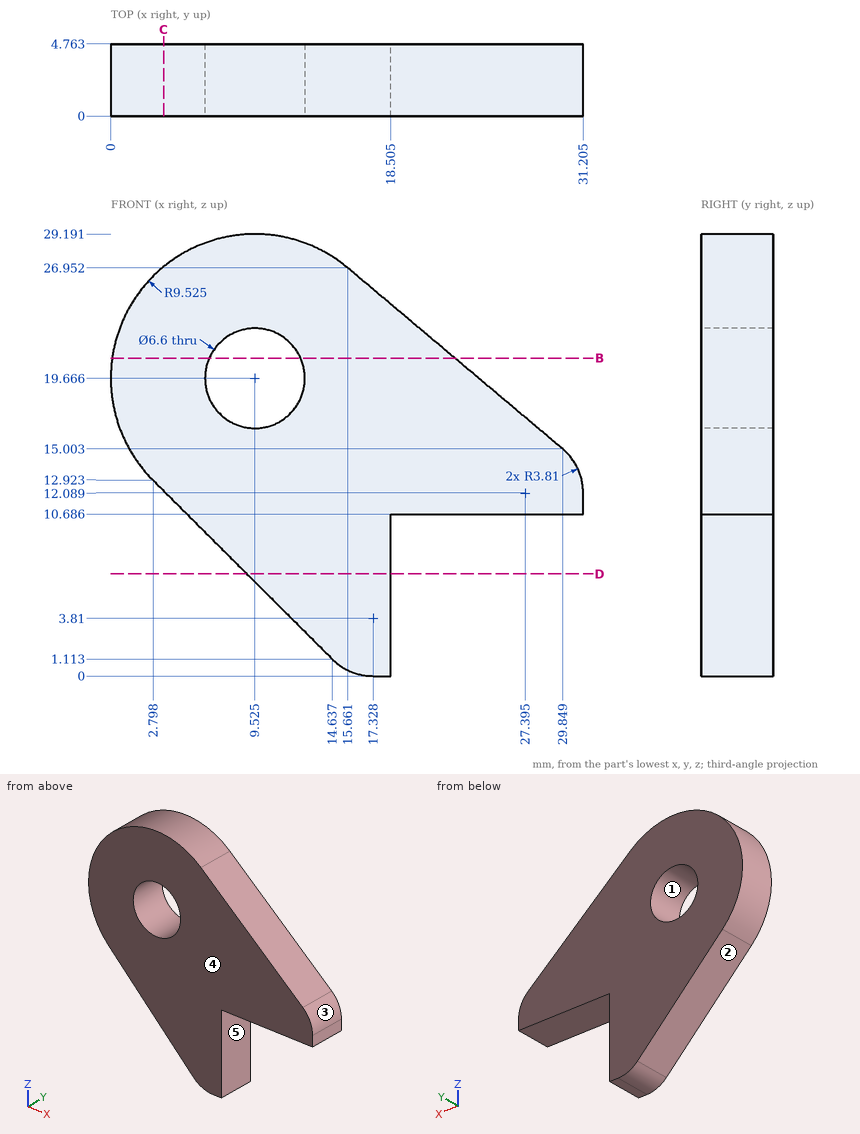
Input: dimensioned drawing with shaded views. Units: mm. Origin: part minimum x, y, z. A direction names the side the tool comes from. Coordinates: 2 decimals unless noted, no trailing zeros. Loops run counter-clockwise (first coordinate to the right, second up) from the corner with the lowest first, then second, coordinate; pieces in that order, holes last. Notation, with made-up numbers: M 89.5,30.25 L 116.5,30.25 A21 ccw 116.5,60.25 Z; hole C 86,-15.5 d9. An arc over 180 degrees is marked long. Use a Markdown table: item, result. Add a question column.
Q1. Section query C-C, the plane x = 3.5. Return loops of the section in (y, z).
Q2. Section query D-D, the plane z = 6.75. Return loops of the section in (x, y) (1 decimal).
Q3. First-contact query: pin 1 (4 mm diameter, centred on x = 9.52, z = 19.67, fed in from -Y); pin 2 (1.5 mm diameter, centred on y = 3, z = 18.5, fed in from -X); pin 3 (2 mm diameter, centred on y = 1.5, z = 11.5, fed in from -X); pin 4 (2.5 mm diameter, centred on x = 23, y = 3, fed in from -Z). Flat tips, straight axial feed; report the tip coordinate or a pass-through.
Q4. Section query B-B, the plane z = 21. Return loops of the section in (x, y).
Q5. Access query for the marked faces 4 and 5. Directions: +Z, -Z, +X, -X, +Y, -Y. A direction counts if a zero-diameter tool reaches every point of the face in a straight line with its end or side. Return the directions, or none.
Q6. Draft query along X for the marked faces 1, 2 and 3. Return one class per face: pulls with the +X half, pulls with the -X half, needs draft (parallel to the pull), parting line crosses it, or undercut.
Q7. Material intervals for L1, parallel to Z at x = 7.5, y = 1.85 (1 decimal); L2, parallel to Z at x = 9, y = 1.8 (1 decimal); L3, parallel to X at y = 3.8, z = 20 (1 decimal), sorted ascending.
Result:
| question | item | result |
|---|---|---|
| 1 | outline | M 0,12.22 L 4.76,12.22 L 4.76,27.04 L 0,27.04 Z |
| 2 | outline | M 9,0 L 18.5,0 L 18.5,4.8 L 9,4.8 Z |
| 3 | pin 1 | passes through |
| 3 | pin 2 | stops at x = 0.01 |
| 3 | pin 3 | stops at x = 3.22 |
| 3 | pin 4 | stops at z = 10.69 |
| 4 | outline | M 0.09,0 L 6.51,0 L 6.51,4.76 L 0.09,4.76 Z; M 12.54,0 L 22.73,0 L 22.73,4.76 L 12.54,4.76 Z |
| 5 | face 4 | +Z, -Z, +X, -X, -Y |
| 5 | face 5 | -Z, +X, +Y, -Y |
| 6 | face 1 | undercut |
| 6 | face 2 | pulls with the -X half |
| 6 | face 3 | pulls with the +X half |
| 7 | L1 | z = 8.2 to 17.1, 22.3 to 29 |
| 7 | L2 | z = 6.7 to 16.4, 22.9 to 29.2 |
| 7 | L3 | x = 0 to 6.2, 12.8 to 23.9 |
